```python
from build123d import *

# Parameters (mm, degrees)
SKETCH_1_R             = 9.75
EXTRUDE_1_DEPTH        = 3
SKETCH_2_R             = 5.25
EXTRUDE_2_DEPTH        = 1.8
SKETCH_3_R             = 2.5
CUT_EXTRUDE_1_DEPTH    = 3.7
HOLE_WIZARD_M3_1_D     = 2.5
HOLE_WIZARD_M3_1_DEPTH = 8.5
HOLE_WIZARD_M3_1_TIP   = 0.751075774
SKETCH_10_R            = 1.5
CUT_EXTRUDE_2_DEPTH    = 3.7


with BuildPart() as part:
    # 草图1 → 凸台-拉伸1 (new body)
    with BuildSketch(Plane(origin=(0, 0, 0), x_dir=(1, 0, 0), z_dir=(0, 1, 0))):
        with Locations(Location((0, 0, 0), (0, 0, 270))):
            Circle(SKETCH_1_R)
    extrude(amount=EXTRUDE_1_DEPTH)

    # 草图2 → 凸台-拉伸2 (add)
    with BuildSketch(Plane(origin=(0, 3, 0), x_dir=(1, 0, 0), z_dir=(0, 1, 0))):
        with Locations(Location((0, 0, 0), (0, 0, 270))):
            Circle(SKETCH_2_R)
    extrude(amount=EXTRUDE_2_DEPTH)

    # 草图3 → 切除-拉伸1 (cut)
    with BuildSketch(Plane(origin=(0, 4.8, 0), x_dir=(1, 0, 0), z_dir=(0, 1, 0))):
        with Locations(Location((0, 0, 0), (0, 0, 270))):
            Circle(SKETCH_3_R)
    extrude(amount=-CUT_EXTRUDE_1_DEPTH, mode=Mode.SUBTRACT)

    # M3 螺纹孔1
    with Locations(Plane(origin=(0, 3, 0), x_dir=(1, 0, 0), z_dir=(0, 1, 0))):
        with Locations((0, 7), (7, 0), (0, -7), (-7, 0)):
            Hole(HOLE_WIZARD_M3_1_D / 2, depth=HOLE_WIZARD_M3_1_DEPTH)
            with Locations((0, 0, -(HOLE_WIZARD_M3_1_DEPTH + HOLE_WIZARD_M3_1_TIP / 2))):  # 118° drill point
                Cone(0, HOLE_WIZARD_M3_1_D / 2, HOLE_WIZARD_M3_1_TIP, mode=Mode.SUBTRACT)

    # 草图10 → 切除-拉伸2 (cut)
    with BuildSketch(Plane(origin=(0, 1.1, 0), x_dir=(1, 0, 0), z_dir=(0, 1, 0))):
        with Locations(Location((0, 0, 0), (0, 0, 270))):
            Circle(SKETCH_10_R)
    extrude(amount=-CUT_EXTRUDE_2_DEPTH, mode=Mode.SUBTRACT)


solid = part.part
```
For this review, take the finished solid that the model builds, in its own axes (mm). A direction names the side the tool comes from. Round coordinates to 2 decimals unless told otherwise and drop trailing zeros. Write each loop counter-clockwise with the first axis right and the second up, starting at its lowest first coordinate (ties: lowest second). Pieces come first, ordered by that corner, then holes. Notation, with made-up numbers: (73, -34) -> (131, -34) arc R33 cw to (131, 3) -> close; hole circle Ø7 at (6.5, 44). An arc over 180 degrees is marked (long way). Use one line per item in the form item = value.
Q1. Consider section A-A (x = 0). State the section outline as (y, z) points, then the cut area to 3 significant figures.
Resolved:
outline = (0, -9.75) -> (3, -9.75) -> (3, -8.25) -> (0, -8.25) -> close; (0, -5.75) -> (3, -5.75) -> (3, -5.25) -> (4.8, -5.25) -> (4.8, -2.5) -> (1.1, -2.5) -> (1.1, -1.5) -> (0, -1.5) -> close; (0, 1.5) -> (1.1, 1.5) -> (1.1, 2.5) -> (4.8, 2.5) -> (4.8, 5.25) -> (3, 5.25) -> (3, 5.75) -> (0, 5.75) -> close; (0, 8.25) -> (3, 8.25) -> (3, 9.75) -> (0, 9.75) -> close
area = 40.6 mm²
Q2. The part is to be moulded in two halves that separate along X. For faces 3 (the cylindrical face through (-5.75, 1.48, -0.05)), 4 (the flat face through (-4, 3, 4)), 5 (the cylindrical face through (9.667, 1.479, -1.269)), say which applies: released by +X, released by -X, zero draft, split by the parting line, or undercut.
Resolved:
face_3 = undercut
face_4 = zero draft
face_5 = split by the parting line
Q3. Consider section D-D (x = 7). State the section outline as (y, z) points, then the cut area to 3 significant figures.
Resolved:
outline = (0, -6.79) -> (3, -6.79) -> (3, -1.25) -> (0, -1.25) -> close; (0, 1.25) -> (3, 1.25) -> (3, 6.79) -> (0, 6.79) -> close
area = 33.2 mm²
Q4. Consider section B-B (y = 0.5). State the section outline as (x, z) points, then the cut area to 3 significant figures.
Resolved:
outline = circle Ø19.5 at (0, 0); hole circle Ø2.5 at (-7, 0); hole circle Ø3 at (0, 0); hole circle Ø2.5 at (0, -7); hole circle Ø2.5 at (0, 7); hole circle Ø2.5 at (7, 0)
area = 272 mm²
Q5. Consider section C-C (z = -0.25). State the section outline as (x, y) points.
Resolved:
outline = (-9.75, 0) -> (-8.22, 0) -> (-8.22, 3) -> (-9.75, 3) -> close; (-5.78, 0) -> (-1.48, 0) -> (-1.48, 1.1) -> (-2.49, 1.1) -> (-2.49, 4.8) -> (-5.24, 4.8) -> (-5.24, 3) -> (-5.78, 3) -> close; (1.48, 0) -> (5.78, 0) -> (5.78, 3) -> (5.24, 3) -> (5.24, 4.8) -> (2.49, 4.8) -> (2.49, 1.1) -> (1.48, 1.1) -> close; (8.22, 0) -> (9.75, 0) -> (9.75, 3) -> (8.22, 3) -> close
Q6. To check wall thickness, follow probe 1 along X at (y, z) = (1.85, 0.25); probe 2 along X at (y, z) = (1.45, -0.5); probe 3 along Y at (x, z) = (2.25, -0.5). State the ranges of each line that lie inside material, in increasing order. Write a range as from..to.
Resolved:
probe_1 = -9.75..-8.22, -5.78..-2.49, 2.49..5.78, 8.22..9.75
probe_2 = -9.74..-8.15, -5.85..-2.45, 2.45..5.85, 8.15..9.74
probe_3 = 0..1.1
Q7. Machinability: for faces 1 (the cylindrical face through (-2.44, 2.98, -0.54)), 2 (the cylindrical face through (0.45, 0.56, 1.43)), which of the approach directions +Z, -Z, +X, -X, +Y, -Y give a long, thin tool a straight path to every point of the face, cutting with its end or side? Answer none if there is none.
Resolved:
face_1 = +Y
face_2 = +Y, -Y
Q8. Clearance check with flat-ended pins moving along their axes: pin 1 Ø1.5 at (x, y) = (2, 3) entering from +Z; pin 2 Ø2 at (x, y) = (-4, 2.5) entering from +Z; pin 3 Ø2.5 at (x, z) = (0, 0) entering from +Y; pin 4 Ø1.5 at (x, z) = (-0.5, 1) entering from +Y. State where each tip first meets the part, or that it passes through.
Resolved:
pin_1 = 9.67
pin_2 = 9.28
pin_3 = through
pin_4 = 1.1
